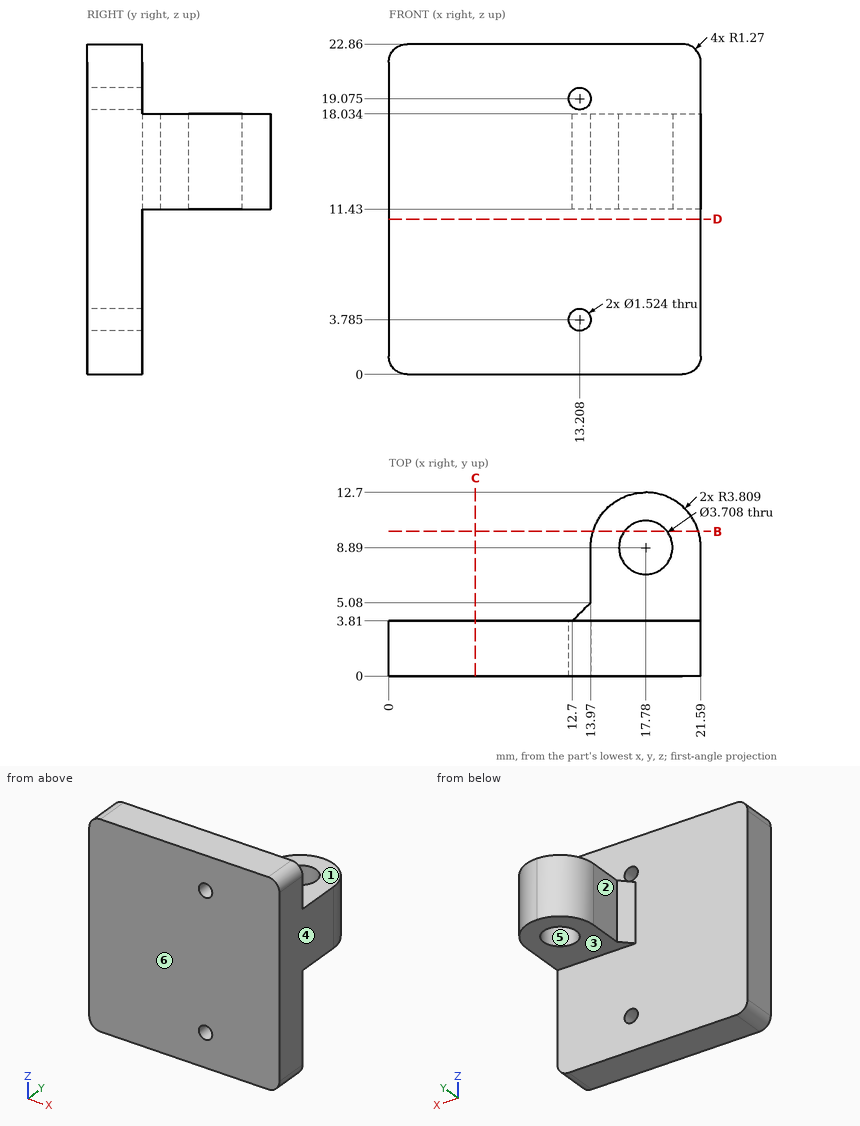
Part print with two shaded views. Sizes in mm from the minimum x, y, z corner. A direction names the side the tool comes from. Give positions to 0.01 mm unless a question says otherwise; leave off trailing zeros. Order: outer loops, then holes, each group sorted by start corner. A loop starts at its lowest first (then second) coordinate and runs counter-clockwise, first axis right, second up.
1) Pin check, flat tips, straight feed: pin 1 (6 mm diameter, centred on x = 15, y = 8.5, fed in from -Z); pin 2 (1 mm diameter, centred on y = 6.5, z = 16.5, fed in from -X); pin 3 (4 mm diameter, centred on x = 15.5, z = 12.5, fed in from +Y). Stop position of each tip, or through.
2) Mould opens along X. For the marked faces 4, 5 and 6 say: +X half, -X half, draft (parallel to the pull), parting line (faces both ways), or undercut.
3) 3-axis set-ups, long thin cutter, end or side, ignore diameter. For the marked faces 1, 2 and 3: which of +Z, -Z, +X, -X, +Y, -Y reach the whole face in a straight line?
4) Wall check: probe 1 along Y at (x, z) = (6.25, 17.25); probe 2 along Z at (x, y) = (15.5, 6) (1 decimal); probe 3 along Y at (x, z) = (13.5, 14). Give the ranges that are in metal, low to high.
5) Saw through at B-B, the plane y = 10. Write the cut outline in (x, z) (1 decimal).
6) Saw through at D-D, the plane z = 10.75. Write the cut outline in (x, y).
7) Saw through at C-C, the plane x = 6. Write the cut outline in (y, z).
Computed:
1. pin 1: stops at z = 11.43
1. pin 2: stops at x = 13.97
1. pin 3: stops at y = 12.69
2. face 4: +X half
2. face 5: undercut
2. face 6: draft
3. face 1: +Z, +X, -X, +Y
3. face 2: +Z, -Z, -X, +Y
3. face 3: -Z, +X, -X, +Y
4. probe 1: y = 0 to 3.81
4. probe 2: z = 11.4 to 18
4. probe 3: y = 0 to 4.61
5. outline: (14.1, 11.4) - (16.3, 11.4) - (16.3, 18) - (14.1, 18) - close; (19.3, 11.4) - (21.4, 11.4) - (21.4, 18) - (19.3, 18) - close
6. outline: (0, 0) - (21.59, 0) - (21.59, 3.81) - (0, 3.81) - close
7. outline: (0, 0) - (3.81, 0) - (3.81, 22.86) - (0, 22.86) - close
